Geometry check sheet. Reference: the model listing, model coordinates, mm. A direction names the side the tool comes from. Give positions to 0.01 mm unless a question says otherwise; leave off trailing zeros. Order: outer loops, then holes, each group sorted by start corner. A loop starts at its lowest first (then second) coordinate and runs counter-clockwise, first axis right, second up. Notation, with made-up numbers: M 11.25,12.25 L 46.25,12.25 A30 ccw 46.25,36.25 Z; hole C 82,63.5 d9. An arc over 180 degrees is marked long. Answer as CSV lines item,"result". Start each with the question number.
Autodesk Inventor part; units mm, degrees
ref_plane "YZ Plane" through (0, 0, 0) normal (1, 0, 0) x (0, 1, 0)
ref_plane "XZ Plane" through (0, 0, 0) normal (0, 1, 0) x (-1, 0, 0)
ref_plane "XY Plane" through (0, 0, 0) normal (0, 0, 1) x (1, 0, 0)
sketch "Sketch1" plane through (0, 0, 0) normal (0, 1, 0) x (-1, 0, 0)
  line L0 (38.8889, 27.7778) -> (-11.1111, 27.7778)
  line L1 (-11.1111, 27.7778) -> (-11.1111, -22.2222)
  line L2 (38.8889, 27.7778) -> (38.8889, 22.7778)
  line L3 (38.8889, 22.7778) -> (-6.1111, 22.7778)
  line L4 (-6.1111, 22.7778) -> (-6.1111, -22.2222)
  line L5 (-6.1111, -22.2222) -> (-11.1111, -22.2222)
  point P0 (0, 0)
  dimension "d0" = 50
  dimension "d1" = 50
  dimension "d2" = 5
  dimension "d3" = 5
extrude "Extrusion1" add sketch "Sketch1" along normal blind 1000
properties part number "Ugol800" material "Aluminum 6061"
Item 1: Scan lines: line 1 along X through (y, z) = (111.5, 18.5); line 2 along Z through (x, y) = (-35, 647). Record each from-to range of solid material in increasing order.
Item 2: Section check B-B on y = 612.5. Record the boundary of the cut face in (x, z), then the cut area to 3 significant figures.
Item 3: Access from +Z, -Z, +X, -X, +Y, -Y to the whole of each face (thin tool, end or side, straight path). Record for faces 1 (the face through (7, 0, 14)), 2 (the face through (-17, 493, 22.778)).
Item 4: Section check C-C on z = 4.5. Record the boundary of the cut face in (x, y).
Item 5: Depth check by flat-ended pin: pin 1 Ø13.5 at (y, z) = (336.5, -8.5) entering from -X. Enter the tip coordinate at first touch or a pass-through.
Item 6: Section check A-A on x = -5. Record the boundary of the cut face in (y, z).
Numbers:
1,line 1,"6.11 to 11.11"
1,line 2,"22.78 to 27.78"
2,outline,"M -38.89,22.78 L 6.11,22.78 L 6.11,-22.22 L 11.11,-22.22 L 11.11,27.78 L -38.89,27.78 Z"
2,area,"475 mm2"
3,face 1,"+Z, -Z, +X, -X, -Y"
3,face 2,"-Z, -X, +Y, -Y"
4,outline,"M 6.11,0 L 11.11,0 L 11.11,1000 L 6.11,1000 Z"
5,pin 1,"x = 6.11"
6,outline,"M 0,22.78 L 1000,22.78 L 1000,27.78 L 0,27.78 Z"
